The listing builds one solid part. Answer for the finished solid, in the listing's coordinates (mm). Face numbers are marked on the shaded views. A direction names the side the tool comes from. Coordinates: 2 decimals unless noted, no trailing zeros. Order: outer loops, then holes, each group sorted by start corner. A loop starts at its lowest first (then second) coordinate and runs counter-clockwise, first axis right, second up. Notation, with made-up numbers: (-17, 47) -> (9, 47) arc R24 cw to (9, 70) -> close; hole circle Ø10 at (85, 80). An arc over 180 degrees is marked (long way). Return JSON: item names as keys, results as strings.
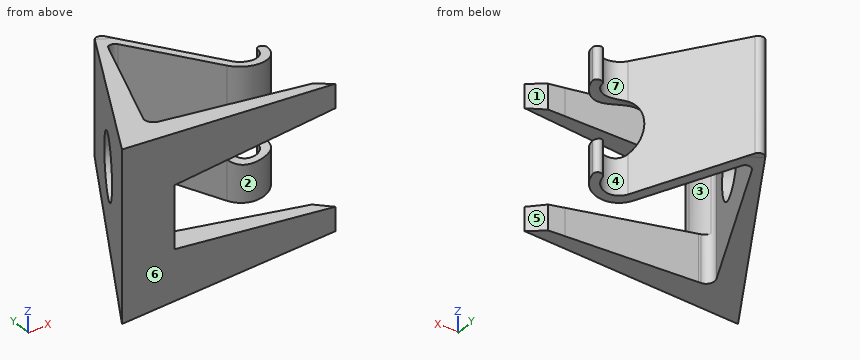
```python
from build123d import *

# Parameters (mm, degrees)
F1_DEPTH      = 58
F3_DEPTH      = 25
F5_DEPTH      = 95.4
F6_R          = 15
F7_R          = 10
F8_DEPTH      = 10
F8_DEPTH_BACK = 20
F9_R          = 10.4169044955
F10_DEPTH     = 25


with BuildPart() as f1:
    # F0 (on Top) → F1 (new body)
    with BuildSketch(Plane.XY):
        with BuildLine():
            ThreePointArc((11.3887710857, 47.9319766204), (9.6390886527, 48.9631570378), (7.8894062197, 47.9319766204))
            Line((7.8894062197, 47.9319766204), (-27.7575390254, -16.4461955428))
            Line((-27.7575390254, -16.4461955428), (45.5045364797, -16.4461955428))
            Line((45.5045364797, -16.4461955428), (40.2530199854, -12.4482339651))
            Line((40.2530199854, -12.4482339651), (34.8717773227, -11.8983741444))
            Line((34.8717773227, -11.8983741444), (-7.9129768242, -7.5265926221))
            Line((-7.9129768242, -7.5265926221), (-8.7686574365, -7.4391584702))
            ThreePointArc((-8.7686574365, -7.4391584702), (-11.0484779416, -5.9775041051), (-11.2219896129, -3.2749296438))
            Line((-11.2219896129, -3.2749296438), (7.8894062197, 41.407315159))
            ThreePointArc((7.8894062197, 41.407315159), (9.6390886527, 42.4384955764), (11.3887710857, 41.407315159))
            Line((11.3887710857, 41.407315159), (27.8816032063, 11.6213579495))
            ThreePointArc((27.8816032063, 11.6213579495), (37.1870634085, 7.3303350671), (44.0722971617, 14.9196712118))
            ThreePointArc((44.0722971617, 14.9196712118), (42.6641613212, 16.6551483551), (40.9286841779, 15.2470125146))
            ThreePointArc((40.9286841779, 15.2470125146), (36.556153133, 10.4273347675), (30.6466350134, 13.1523883301))
            Line((30.6466350134, 13.1523883301), (11.3887710857, 47.9319766204))
        make_face()
    extrude(amount=F1_DEPTH)

    # F2 (on face) → F3 (cut)
    with BuildSketch(Plane(origin=(-0.842891654, -8.2490197652, 0), x_dir=(-0.9948200667, 0.1016515362, 0), z_dir=(0.1016515362, 0.9948200667, 0))):
        Polygon((-41.3098941341, 13.2178132166), (-41.3098941341, 29), (-83.8253051043, 29), (-83.8253051043, 8.7828920186), align=None)
        Polygon((-41.3098941341, 29), (-41.3098941341, 44.7821867834), (-83.8253051043, 49.2171079814), (-83.8253051043, 29), align=None)
        Polygon((7.9670344895, 29), (7.9670344895, 39.6419496238), (-41.3098941341, 44.7821867834), (-41.3098941341, 29), align=None)
        Polygon((7.9670344895, 18.3580503762), (7.9670344895, 29), (-41.3098941341, 29), (-41.3098941341, 13.2178132166), align=None)
    extrude(amount=-F3_DEPTH, mode=Mode.SUBTRACT)

    # F4 (on face) → F5 (cut)
    with BuildSketch(Plane(origin=(-14.2745575957, 7.9039891304, 0), x_dir=(-0.4844097913, -0.8748412165, 0), z_dir=(-0.8748412165, 0.4844097913, 0))):
        Polygon((-45.7545743561, 0), (27.833833402, 0), (-45.7545743561, 9.3257259006), align=None)
        Polygon((-45.7545743561, 58), (-45.7545743561, 48.6742740994), (27.833833402, 58), align=None)
        Polygon((27.833833402, -12.4238803983), (27.833833402, 0), (-45.7545743561, 0), (-45.7545743561, 9.3257259006), (-52.6641197503, 10.201360099), (-53.7899360061, -12.4238803983), align=None)
        Polygon((-52.6641197503, 47.798639901), (-45.7545743561, 48.6742740994), (-45.7545743561, 58), (27.833833402, 58), (27.833833402, 63.3924901485), (-55.1632341309, 67.5189115496), align=None)
    extrude(amount=-F5_DEPTH, mode=Mode.SUBTRACT)

    # F6
    f6_edges = [f1.edges().sort_by_distance(p)[0] for p in [
        (-8.768657, -7.439158, 10.261165),
        (-8.768657, -7.439158, 29),
        (-8.768657, -7.439158, 47.738835),
    ]]
    fillet(f6_edges, radius=F6_R)

    # F7 (on face) → F8 (cut, two sides)
    with BuildSketch(Plane(origin=(29.0290557323, 16.0737269393, 0), x_dir=(-0.4844097913, 0.8748412165, 0), z_dir=(0.8748412165, 0.4844097913, 0))) as f8_sk:
        with Locations((-8.284128271, 29)):
            Circle(F7_R)
    extrude(amount=-F8_DEPTH, mode=Mode.SUBTRACT)
    extrude(f8_sk.sketch, amount=F8_DEPTH_BACK, mode=Mode.SUBTRACT)

    # F9 (on face) → F10 (cut)
    with BuildSketch(Plane(origin=(-14.2745575957, 7.9039891304, 0), x_dir=(-0.4844097913, -0.8748412165, 0), z_dir=(-0.8748412165, 0.4844097913, 0))):
        with Locations((-9.4790859148, 29)):
            Circle(F9_R)
    extrude(amount=-F10_DEPTH, mode=Mode.SUBTRACT)


solid = f1.part
```
Item 1: Flat-ended cylindrical pins translate along their axes: pin 1 (1.5 mm diameter, centred on y = 5.5, z = 50.5, fed in from -X); pin 2 (8 mm diameter, centred on x = -9, z = 10, fed in from +Y); pin 3 (1 mm diameter, centred on x = -2, z = 18.5, fed in from -Y). Find the tip coordinate at first contact, or state that the pin passes through.
Answer list:
{"pin 1": "x = -16.02", "pin 2": "y = 24.65", "pin 3": "y = 17.12"}
Item 2: The part is cut by section A-A on x = 21. Determine the outline of the cut face in (y, z), plus the area to 3 significant figures.
Answer list:
{"outline": "(-16.45, 2.99) -> (-10.48, 3.65) -> (-10.48, 15.24) -> (-16.45, 15.17) -> close; (-16.45, 42.83) -> (-10.48, 42.76) -> (-10.48, 54.35) -> (-16.45, 55.01) -> close; (24.05, 7.48) -> (30.57, 8.21) -> (30.57, 49.79) -> (24.05, 50.52) -> close", "area": "418 mm2"}
Item 3: Determine the mould class of the marked faces 5, 6 and 7 for opening direction Y: pulls with the +Y half, pulls with the -Y half, needs draft (parallel to the pull), parting line crosses it, or undercut.
Answer list:
{"face 5": "undercut", "face 6": "pulls with the -Y half", "face 7": "pulls with the +Y half"}
Item 4: The part is cut by section C-C on z = 23.5. Determine the outline of the cut face in (x, y).
Answer list:
{"outline": "(-27.76, -16.45) -> (-9.69, -16.45) -> (-9.48, -14.35) arc R15 ccw to (-11.12, -5.85) arc R3 cw to (-11.22, -3.27) -> (-7.69, 4.98) -> (-13.97, 8.46) -> close; (-5.4, 23.94) -> (-0.7, 21.33) -> (7.89, 41.41) arc R2 cw to (11.39, 41.41) -> (26.23, 14.6) -> (29, 16.13) -> (11.39, 47.93) arc R2 ccw to (7.89, 47.93) -> close"}
Item 5: The part is cut by section B-B on y = 39. Determine the outline of the cut face in (x, z), plus the area to 3 significant figures.
Answer list:
{"outline": "(2.94, 8.03) -> (6.86, 8.27) -> (6.86, 49.73) -> (2.94, 49.97) -> close; (12.72, 8.63) -> (16.33, 8.85) -> (16.33, 49.15) -> (12.72, 49.37) -> close", "area": "310 mm2"}
Item 6: Find the intervals of material crossed by probe 1 along Y at (x, z) = (30.5, 6); probe 2 along Y at (x, z) = (-3, 49); probe 3 along Y at (x, z) = (-5, 50.5), in increasing order.
Answer list:
{"probe 1": "-16.45 to -11.45", "probe 2": "-16.45 to -8.03, 15.95 to 28.27", "probe 3": "-16.45 to -7.82, 11.27 to 24.65"}
Item 7: Which of the six approach directions +Z, -Z, +X, -X, +Y, -Y give full straight-line access (tool end or side, diameter ignored) to the marked faces 1, 2, 3 and 4?
Answer list:
{"face 1": "+Z, -Z, +X", "face 2": "+Z, -Z", "face 3": "+X", "face 4": "+Z, -Z, +Y"}
Item 8: The part is cut by section D-D on x = 36.5. Count the separate pieces of the cut face and the enclosed holes in it, plus the area to 3 significant figures.
Answer list:
{"separate pieces": "4", "enclosed holes": "0", "area": "162 mm2"}
